Study the drawing (mm; zero at the part's minimum x, y, z) and answer. Coordinates: 2 decimals unless noted, no trailing zeros. Order: outer loops, then holes, each group sorted by start corner. A loop starts at its lowest first (then second) coordinate and runs counter-clockwise, first axis right, second up. Notation, with made-up numbers: M 61.5,52 L 110.5,52 A7 ccw 110.5,61 Z; hole C 65,-37.5 d8. An arc over 180 degrees is marked long. Use a Markdown table: item, result. Add a question column.
1) Each of these flat-tipped pins is pushed along its axis until it touches: pin 1 Ø4 at (x, z) = (7.5, 18.5) entering from -Y (1 decimal); pin 2 Ø5 at (x, z) = (5, 7) entering from -Y. Where does it stop, or does it pass through?
2) Find section A-A on z = 6.5. Write down the section's boundary in (x, y).
3) The mould has two halves that part along Y. Classify the marked faces 1, 2 and 3: released by +Y, released by -Y, zero draft, split by the parting line, or undercut.
4) Find the intervals of material crossed by probe 1 along Y at (x, z) = (4.25, 7.5); probe 2 along Z at (x, y) = (5, 6); probe 3 along X at (y, z) = (4, 14) (1 decimal), in increasing order. Write a range as [from, to].
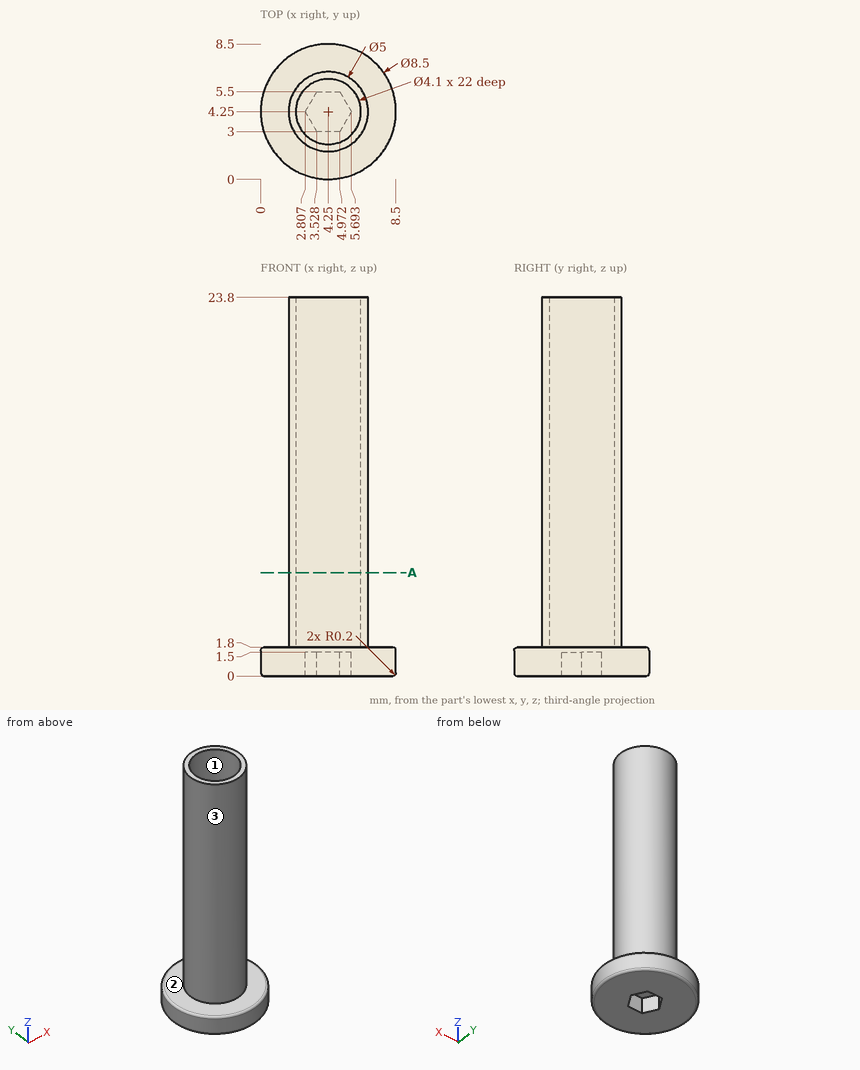
Check result:
| question | item | result |
|---|---|---|
| 1 | pin 1 | stops at y = 2.1 |
| 1 | pin 2 | stops at y = 1.75 |
| 2 | outline | C 4.25,4.25 d5; hole C 4.25,4.25 d4.1 |
| 3 | face 1 | undercut |
| 3 | face 2 | zero draft |
| 3 | face 3 | split by the parting line |
| 4 | probe 1 | y = [1.75, 2.2], [6.3, 6.75] |
| 4 | probe 2 | z = [0, 1.8] |
| 4 | probe 3 | x = [1.8, 2.2], [6.3, 6.7] |
